Geometry: final body of the model. Coordinates: model frame, mm. Face numbers are marked on the shaded views. A direction names the side the tool comes from. Round coordinates to 2 decimals unless told otherwise and drop trailing zeros. Loops run counter-clockwise (first coordinate to the right, second up) from the corner with the lowest first, then second, coordinate; pieces in that order, holes last. Notation, with made-up numbers: (38.5, 42) - (43.5, 42) arc R8 ccw to (43.5, 51) - close; hole circle Ø11 at (-10, 39). An arc over 180 degrees is marked (long way). Write item = value, one per line. Start each with the question number.
Item 1: Access query for the marked faces 4, 5 and 6. Directions: +Z, -Z, +X, -X, +Y, -Y. A direction counts if a zero-diameter tool reaches every point of the face in a straight line with its end or side. Return the directions, or none.
Item 2: Section D-D (z = -4.25). Return loops of the section in (x, y) (3 decimals).
Item 3: First-contact query: pin 1 (3 mm diameter, centred on x = 18, z = -7.5, fed in from +Y); pin 2 (5.5 mm diameter, centred on y = 9.5, z = -14, fed in from -X); pin 3 (10 mm diameter, centred on y = 16.5, z = -5, fed in from +X); pin 4 (1.9 mm diameter, centred on x = 23, z = -10.5, fed in from +Y) (1 decimal). Flat tips, straight axial feed; report the tip coordinate or a pass-through.
Item 4: Section B-B (x = 5). Return loops of the section in (y, z), plus the area to 3 significant figures.
Item 5: Line query: line 1 (X direction, y = 20.5, z = -17); line 2 (Y direction, x = 23.25, z = -5.5); line 3 (X direction, y = 2.5, z = -9.75). Output: solid intervals per line, ascending. Write a range as from..to.
Item 6: Section C-C (y = 19). Return loops of the section in (x, z), plus the area to 3 significant figures.
Item 7: Section A-A (z = -7.75). Return loops of the section in (x, y) (3 decimals).
Item 8: Draft query along X for the marked faces 1, 2 and 3. Return one class per face: pulls with the +X half, pulls with the -X half, needs draft (parallel to the pull), parting line crosses it, or undercut.
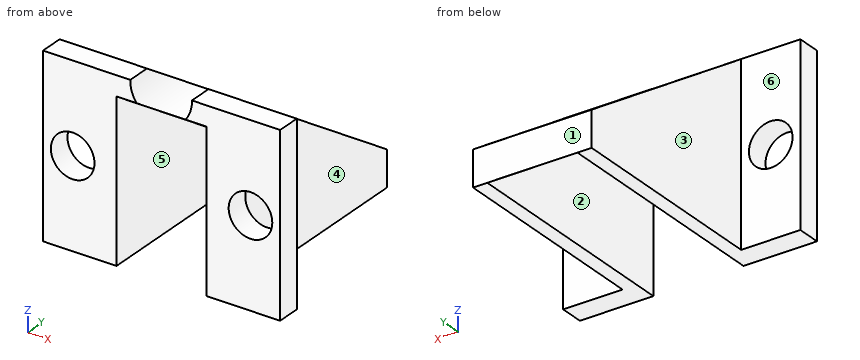
from build123d import *

# Parameters (mm, degrees)
SKETCH1_W           = 25.4
SKETCH1_H           = 19.05
BOSS_EXTRUDE1_DEPTH = 25.4
CHAMFER1_SIZE       = 22.86
CHAMFER1_SIZE2      = 15.24
SKETCH2_W           = 6.35
SKETCH2_H           = 22.78915262
CUT_EXTRUDE1_DEPTH  = 22.86
SKETCH3_W           = 9.652
SKETCH3_H           = 39.353766532
CUT_EXTRUDE2_DEPTH  = 22.86
SKETCH4_R           = 2.3368
CUT_EXTRUDE3_DEPTH  = 22.86
SKETCH6_R           = 3.302
CUT_EXTRUDE5_DEPTH  = 26.4


with BuildPart() as part:
    # Sketch1 → Boss-Extrude1 (new body)
    with BuildSketch(Plane(origin=(0, 0, 0), x_dir=(1, 0, 0), z_dir=(0, 1, 0))):
        with Locations((12.7, 9.525)):
            Rectangle(SKETCH1_W, SKETCH1_H)
    extrude(amount=BOSS_EXTRUDE1_DEPTH)

    # Chamfer1
    chamfer1_edges = [part.edges().sort_by_distance(p)[0] for p in [
        (12.7, 25.4, 0),
    ]]
    chamfer1_side = [part.faces().sort_by_distance(p)[0] for p in [
        (12.7, 12.7, 0),
    ]]
    chamfer(chamfer1_edges, length=CHAMFER1_SIZE, length2=CHAMFER1_SIZE2, reference=chamfer1_side[0])

    # Sketch2 → Cut-Extrude1 (cut)
    with BuildSketch(Plane(origin=(0, 25.4, 0), x_dir=(1, 0, 0), z_dir=(0, 1, 0))):
        with Locations((22.225, 7.65542369)):
            Rectangle(SKETCH2_W, SKETCH2_H)
        with Locations((3.175, 7.65542369)):
            Rectangle(SKETCH2_W, SKETCH2_H)
    extrude(amount=-CUT_EXTRUDE1_DEPTH, mode=Mode.SUBTRACT)

    # Sketch3 → Cut-Extrude2 (cut)
    with BuildSketch(Plane(origin=(0, -0.979634661, -1.469451992), x_dir=(1, 0, 0), z_dir=(0, 0.554700196, 0.832050294))):
        with Locations((12.7, 14.647750361)):
            Rectangle(SKETCH3_W, SKETCH3_H)
    extrude(amount=-CUT_EXTRUDE2_DEPTH, mode=Mode.SUBTRACT)

    # Sketch4 → Cut-Extrude3 (cut)
    with BuildSketch(Plane(origin=(0, 2.54, 0), x_dir=(1, 0, 0), z_dir=(0, 1, 0))):
        with Locations((3.175, 9.525)):
            Circle(SKETCH4_R)
        with Locations((22.225, 9.525)):
            Circle(SKETCH4_R)
    extrude(amount=-CUT_EXTRUDE3_DEPTH, mode=Mode.SUBTRACT)

    # Sketch6 → Cut-Extrude5 (cut, through all)
    with BuildSketch(Plane.XZ):
        with Locations((12.652625, -0.124494929)):
            Circle(SKETCH6_R)
    extrude(amount=-CUT_EXTRUDE5_DEPTH, mode=Mode.SUBTRACT)


solid = part.part
Taken from the geometry:
q1.face_4 = +Z, -Z, +X, +Y
q1.face_5 = -Z, -Y
q1.face_6 = +Z, -Z, -X, +Y
q2.outline = (0, 0) - (7.874, 0) - (7.874, 3.191) - (17.526, 3.191) - (17.526, 0) - (25.4, 0) - (25.4, 2.54) - (19.05, 2.54) - (19.05, 8.915) - (6.35, 8.915) - (6.35, 2.54) - (0, 2.54) - close
q3.pin_1 = 16.04
q3.pin_2 = 6.35
q3.pin_3 = 19.05
q3.pin_4 = through
q4.outline = (0, -19.05) - (2.54, -19.05) - (2.54, -10.98) - (0, -10.98) - close; (0, -8.07) - (2.54, -8.07) - (2.54, 0) - (0, 0) - close
q4.area = 41.0 mm^2
q5.line_1 = 6.35..7.87, 17.53..19.05
q5.line_2 = 0..2.54
q5.line_3 = 0..0.85, 5.5..7.87, 17.53..19.9, 24.55..25.4
q6.outline = (6.35, -19.05) - (7.87, -19.05) - (7.87, -14.79) - (17.53, -14.79) - (17.53, -19.05) - (19.05, -19.05) - (19.05, -10.97) - (6.35, -10.97) - close
q6.area = 61.4 mm^2
q7.outline = (0, 0) - (1.655, 0) - (1.655, 2.54) - (0, 2.54) - close; (4.695, 0) - (7.874, 0) - (7.874, 8.441) - (17.526, 8.441) - (17.526, 0) - (20.705, 0) - (20.705, 2.54) - (19.05, 2.54) - (19.05, 14.165) - (6.35, 14.165) - (6.35, 2.54) - (4.695, 2.54) - close; (23.745, 0) - (25.4, 0) - (25.4, 2.54) - (23.745, 2.54) - close
q8.face_1 = needs draft
q8.face_2 = undercut
q8.face_3 = pulls with the -X half
